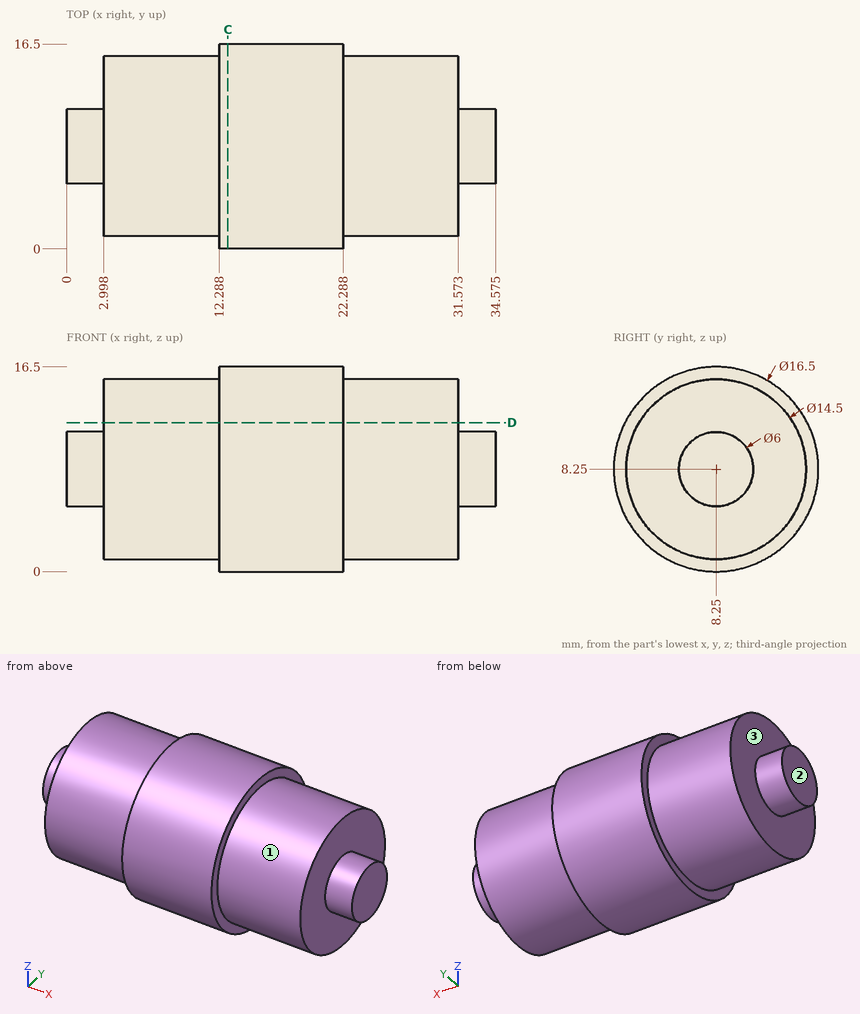
Check sheet for the drawn part. Datum: minimum x, y, z corner. Units: mm. A direction names the side the tool comes from. Give positions to 0.01 mm unless a question says otherwise; leave off trailing zeros. Write each loop counter-clockwise with the first axis right and the second up, starting at its lowest first coordinate (ties: lowest second). Pieces come first, ordered by that corner, then holes. Notation, with made-up numbers: (12, 23.5) -> (58, 23.5) arc R8 ccw to (58, 34.5) -> close; hole circle Ø3 at (-6, -34). An arc over 180 degrees is marked (long way). Use one line per item in the form item = value. Start each with the question number.
1. Access from +Z, -Z, +X, -X, +Y, -Y to the whole of each face (thin tool, end or side, straight path). Record for the marked faces 1, 2 and 3.
2. Section check D-D (z = 12). Record the cut outline in (x, y) (1 decimal).
3. Go/stop test with flat-tipped pins: P1, Ø1.5, axis at x = 13, z = 5.5, coming from the +Y side; P2, Ø3, axis at x = 3.5, z = 2, coming from the -Y side; P3, Ø1, axis at x = 6.5, z = 13, coming from the +Y side (1 decimal). Record where each tip stops, or that it passes through.
4. Thickness scan on line 1 along X through (y, z) = (11.75, 10.25); line 2 along X through (y, z) = (7.25, 1); line 3 along Z through (x, y) = (3.5, 2.25). Record the ranges inside material, lowest first. Write a range as from..to.
5. Section check C-C (x = 13). Record the cut outline in (y, z), and give its area (3 significant figures).
Conclusion:
q1.face_1 = +X
q1.face_2 = +Z, -Z, -X, +Y, -Y
q1.face_3 = -X
q2.outline = (3, 2) -> (12.3, 2) -> (12.3, 0.9) -> (22.3, 0.9) -> (22.3, 2) -> (31.6, 2) -> (31.6, 14.5) -> (22.3, 14.5) -> (22.3, 15.6) -> (12.3, 15.6) -> (12.3, 14.5) -> (3, 14.5) -> close
q3.P1 = 16.25
q3.P2 = 2.77
q3.P3 = 14.1
q4.line_1 = 3..31.57
q4.line_2 = 12.29..22.29
q4.line_3 = 4.18..12.32
q5.outline = circle Ø16.5 at (8.25, 8.25)
q5.area = 214 mm²
